Model file for the job. Use its own axes, mm. A direction names the side the tool comes from. Round coordinates to 2 decimals unless told otherwise and drop trailing zeros. Order: outer loops, then holes, each group sorted by start corner. A loop starts at its lowest first (then second) coordinate and runs counter-clockwise, first axis right, second up. Notation, with made-up numbers: (54.5, 82.25) - (96.5, 82.25) arc R10 cw to (96.5, 97.25) - close; hole circle Ø8 at (-22.75, 58). An arc over 180 degrees is marked (long way). Use one line per item in the form item = value.
from build123d import *

# Parameters (mm, degrees)
SKETCH1_W             = 12.7
SKETCH1_H             = 12.7
BOSS_EXTRUDE1_DEPTH   = 114.3
BOSS_EXTRUDE1_2_DEPTH = 114.3
SKETCH2_W             = 12.7
SKETCH2_H             = 12.7
BOSS_EXTRUDE2_DEPTH   = 254
SKETCH3_W             = 101.6
SKETCH3_H             = 12.7
BOSS_EXTRUDE3_DEPTH   = 114.3
SKETCH4_R             = 1.397
CUT_EXTRUDE1_DEPTH    = 12.7
BOSS_EXTRUDE4_DEPTH   = 12.7
CUT_EXTRUDE2_DEPTH    = 12.7
SKETCH7_W             = 63.5
SKETCH7_H             = 83.82
CUT_EXTRUDE3_DEPTH    = 12.7


with BuildPart() as part:
    # Sketch1 → Boss-Extrude1 (new body)
    with BuildSketch(Plane(origin=(0, 0, 0), x_dir=(1, 0, 0), z_dir=(0, 1, 0))):
        with Locations((-120.65, -6.35)):
            Rectangle(SKETCH1_W, SKETCH1_H)
    extrude(amount=BOSS_EXTRUDE1_DEPTH)



with BuildPart() as body_2:
    # Sketch1 → Boss-Extrude1 2 (new body)
    with BuildSketch(Plane(origin=(0, 0, 0), x_dir=(1, 0, 0), z_dir=(0, 1, 0))):
        with Locations((120.65, -6.35)):
            Rectangle(SKETCH1_W, SKETCH1_H)
    extrude(amount=BOSS_EXTRUDE1_2_DEPTH)


with BuildPart() as part_1:
    add(part.part)

    add(body_2.part)  # Boss-Extrude2 merges body 2
    # Sketch2 → Boss-Extrude2 (add)
    with BuildSketch(Plane.ZY.offset(127)):
        with Locations((6.35, 120.65)):
            Rectangle(SKETCH2_W, SKETCH2_H)
    extrude(amount=-BOSS_EXTRUDE2_DEPTH)

    # Sketch3 → Boss-Extrude3 (add)
    with BuildSketch(Plane.XZ.offset(-114.3)):
        with Locations((0, 6.35)):
            Rectangle(SKETCH3_W, SKETCH3_H)
    extrude(amount=BOSS_EXTRUDE3_DEPTH)

    # Sketch4 → Cut-Extrude1 (cut)
    with BuildSketch(Plane(origin=(127, 0, 0), x_dir=(0, 0, -1), z_dir=(1, 0, 0))):
        with Locations((-6.35, 4.445)):
            Circle(SKETCH4_R)
    cut_extrude1 = extrude(amount=-CUT_EXTRUDE1_DEPTH, mode=Mode.SUBTRACT)

    # Mirror1: Cut-Extrude1 across plane
    add(cut_extrude1.mirror(Plane(origin=(0, 0, 0), x_dir=(0, 0, 1), z_dir=(1, 0, 0))), mode=Mode.SUBTRACT)

    # Sketch5 → Boss-Extrude4 (add)
    with BuildSketch(Plane(origin=(0, 0, 0), x_dir=(-1, 0, 0), z_dir=(0, 0, -1))):
        with BuildLine():
            Line((-114.3, 114.3), (-114.3, 101.6))
            ThreePointArc((-114.3, 101.6), (-110.580256121, 110.580256121), (-101.6, 114.3))
            Line((-101.6, 114.3), (-114.3, 114.3))
        make_face()
        with BuildLine():
            Line((-50.8, 114.3), (-63.5, 114.3))
            ThreePointArc((-63.5, 114.3), (-54.519743879, 110.580256121), (-50.8, 101.6))
            Line((-50.8, 101.6), (-50.8, 114.3))
        make_face()
    boss_extrude4 = extrude(amount=-BOSS_EXTRUDE4_DEPTH)

    # Mirror2: Boss-Extrude4 across plane
    add(boss_extrude4.mirror(Plane(origin=(0, 0, 0), x_dir=(0, 0, 1), z_dir=(1, 0, 0))))

    # Sketch6 → Cut-Extrude2 (cut)
    with BuildSketch(Plane(origin=(0, 0, 0), x_dir=(-1, 0, 0), z_dir=(0, 0, -1))):
        with BuildLine():
            Line((-127, 127), (-127, 114.3))
            ThreePointArc((-127, 114.3), (-123.280256121, 123.280256121), (-114.3, 127))
            Line((-114.3, 127), (-127, 127))
        make_face()
    cut_extrude2 = extrude(amount=-CUT_EXTRUDE2_DEPTH, mode=Mode.SUBTRACT)

    # Mirror3: Cut-Extrude2 across plane
    add(cut_extrude2.mirror(Plane(origin=(0, 0, 0), x_dir=(0, 0, 1), z_dir=(1, 0, 0))), mode=Mode.SUBTRACT)

    # Sketch7 → Cut-Extrude3 (cut)
    with BuildSketch(Plane(origin=(0, 0, 0), x_dir=(-1, 0, 0), z_dir=(0, 0, -1))):
        with Locations((0, 66.04)):
            Rectangle(SKETCH7_W, SKETCH7_H)
    extrude(amount=-CUT_EXTRUDE3_DEPTH, mode=Mode.SUBTRACT)


solid = part_1.part
(1) Pull direction Y, two halves, no side cores. Call faces 4 (the face through (-31.75, 65, 6)), 5 (the face through (0, 24.13, 6)), 6 (the face through (110.68, 110.48, 6.26)), 7 (the face through (-127, 58, 6)): released by +Y, released by -Y, zero draft, split by the parting line, or undercut.
Report:
face_4 = undercut
face_5 = undercut
face_6 = released by -Y
face_7 = zero draft
(2) Slice it at B-B on x = 2.5. Give the cut face in (y, z).
Report:
outline = (0, 0) - (24.13, 0) - (24.13, 12.7) - (0, 12.7) - close; (107.95, 0) - (127, 0) - (127, 12.7) - (107.95, 12.7) - close
(3) Tool access for faces 1 (the face through (-83, 114.3, 6)), 2 (the face through (-1, 111, 12.7)), 3 (the face through (0, 107.95, 6)): list every direction of +Z, -Z, +X, -X, +Y, -Y with a clear straight run to the whole face (end or side of a thin tool).
Report:
face_1 = +Z, -Z, -Y
face_2 = +Z, +X, -X, +Y, -Y
face_3 = +Z, -Z
(4) Slice it at C-C on y = 42. Give the cut face in (x, z).
Report:
outline = (-127, 0) - (-114.3, 0) - (-114.3, 12.7) - (-127, 12.7) - close; (-50.8, 0) - (-31.75, 0) - (-31.75, 12.7) - (-50.8, 12.7) - close; (31.75, 0) - (50.8, 0) - (50.8, 12.7) - (31.75, 12.7) - close; (114.3, 0) - (127, 0) - (127, 12.7) - (114.3, 12.7) - close
(5) Slice it at D-D on x = -87. Give the cut face in (y, z), then the cut area to 3 significant figures.
Report:
outline = (114.3, 0) - (127, 0) - (127, 12.7) - (114.3, 12.7) - close
area = 161 mm2
(6) Slice it at A-A on y = 20. Give the cut face in (x, z).
Report:
outline = (-127, 0) - (-114.3, 0) - (-114.3, 12.7) - (-127, 12.7) - close; (-50.8, 0) - (50.8, 0) - (50.8, 12.7) - (-50.8, 12.7) - close; (114.3, 0) - (127, 0) - (127, 12.7) - (114.3, 12.7) - close
(7) Pin check, flat tips, straight feed: pin 1 (2 mm diameter, centred on y = 4.445, z = 6.35, fed in from -X); pin 2 (1.5 mm diameter, centred on x = -67, z = 10.5, fed in from -Y). Stop position of each tip, or through.
Report:
pin_1 = -50.8
pin_2 = 114.3
(8) Probe probe 1 along X at (y, z) = (55, 2.75); probe 2 along X at (y, z) = (17.5, 1); probe 3 along Y at (x, z) = (-3.5, 9.5). List the from-to ranges inside material, lowest first. Write a range as [from, to].
Report:
probe_1 = [-127, -114.3], [-50.8, -31.75], [31.75, 50.8], [114.3, 127]
probe_2 = [-127, -114.3], [-50.8, 50.8], [114.3, 127]
probe_3 = [0, 24.13], [107.95, 127]
